from build123d import *

# Parameters (mm, degrees)
CYLINDER002_R       = 3.8
CYLINDER002_DEPTH   = 15
CYLINDER001_R       = 2
CYLINDER001_DEPTH   = 16
BOX001_W            = 5
BOX001_H            = 20
BOX001_DEPTH        = 12
BOX_W               = 5
BOX_H               = 20
BOX_DEPTH           = 12
BOX_PLACEMENT_ANGLE = 90
CYLINDER_R          = 10
CYLINDER_DEPTH      = 16


with BuildPart() as cilindro002:
    # Cylinder002 → Cylinder002 (new body)
    with BuildSketch(Plane.XY):
        Circle(CYLINDER002_R)
    extrude(amount=CYLINDER002_DEPTH)


with BuildPart() as fusion001:
    # Cylinder001 → Cylinder001 (new body)
    with BuildSketch(Plane.XY):
        Circle(CYLINDER001_R)
    extrude(amount=CYLINDER001_DEPTH)

    # Fusion001: union Cilindro002
    add(cilindro002.part)


with BuildPart() as cubo001:
    # Box001 → Box001 (new body)
    with BuildSketch(Plane(origin=(-2.5, -10, 0), x_dir=(1, 0, 0), z_dir=(0, 0, 1))):
        with Locations((2.5, 10)):
            Rectangle(BOX001_W, BOX001_H)
    extrude(amount=BOX001_DEPTH)


with BuildPart() as fusion:
    # Box → Box (new body)
    with BuildSketch(Plane.XY):
        with Locations((2.5, 10)):
            Rectangle(BOX_W, BOX_H)
    extrude(amount=BOX_DEPTH)


with BuildPart() as fusion_1:
    # Box placement: moved
    add(fusion.part.moved(Location((10, -2.5, 0))).rotate(Axis((10, -2.5, 0), (0, 0, 1)), BOX_PLACEMENT_ANGLE))

    # Fusion: union Cubo001
    add(cubo001.part)


with BuildPart() as esfera:
    # Sphere → Sphere (revolve)
    with BuildSketch(Plane(origin=(0, 0, 3), x_dir=(1, 0, 0), z_dir=(0, -1, 0))):
        with BuildLine():
            ThreePointArc((0, -8), (8, 0), (0, 8))
            Line((0, 8), (0, -8))
        make_face()
    revolve(axis=Axis((0, 0, 3), (0, 0, 1)))


with BuildPart() as cut002:
    # Cylinder → Cylinder (new body)
    with BuildSketch(Plane.XY):
        Circle(CYLINDER_R)
    extrude(amount=CYLINDER_DEPTH)

    # Cut: cut Esfera
    add(esfera.part, mode=Mode.SUBTRACT)

    # Cut001: cut Fusion
    add(fusion_1.part, mode=Mode.SUBTRACT)

    # Cut002: cut Fusion001
    add(fusion001.part, mode=Mode.SUBTRACT)


solid = cut002.part
Read the model definition and answer for the solid it produces. Units are mm, in the model's axes. A direction names the side the tool comes from. Round coordinates to 2 decimals unless told otherwise and drop trailing zeros. Loops run counter-clockwise (first coordinate to the right, second up) from the corner with the lowest first, then second, coordinate; pieces in that order, holes last.
Q1. Which of the six approach directions +Z, -Z, +X, -X, +Y, -Y give full straight-line access (tool end or side, diameter ignored) to faces 1 (the face through (-6, 6, 0)), 2 (the face through (-7, -2.5, 7)), 3 (the face through (2, -2, 15)), 4 (the face through (2.5, -7, 7))?
Q2. Determine the mould class of faces 5 (the face through (-7, 2.5, 7)), 6 (the face through (-2.5, 7, 7)), 7 (the face through (2.5, 7, 7)), 8 (the face through (9.237, -3.83, 7.888)) for opening direction X: released by +X, released by -X, zero draft, split by the parting line, or undercut.
Q3. Each of these flat-tipped pins is pushed along its axis until it touches: pin 1 (4 mm diameter, centred on x = 2.5, z = 14, fed in from -Y); pin 2 (5.5 mm diameter, centred on y = -7.5, z = 8, fed in from -X); pin 3 (7 mm diameter, centred on x = 0, y = 0, fed in from -Z). Where does it stop, or does it pass through?
Q4. Section A-A on z = 11 is taken. Write down the section's boundary in (x, y).
Q5. Consider probe 1 along Y at (x, z) = (0, 15.65); probe 2 along Y at (x, z) = (0, 12.3). Determine where each line is inside the solid, lowest interval first.
Q6. Section D-D on z = 8.5 is taken. Write down the section's boundary in (x, y).
Q7. Section B-B on x = 0 is taken. Write down the section's boundary in (y, z), and give its area (3 significant figures).
Output:
1. face 1: -Z, +X, -X, +Y, -Y
1. face 2: -Z, +X, -X
1. face 3: -Z
1. face 4: -Z, +Y, -Y
2. face 5: zero draft
2. face 6: undercut
2. face 7: undercut
2. face 8: split by the parting line
3. pin 1: stops at y = -9.99
3. pin 2: stops at x = -8.8
3. pin 3: stops at z = 15
4. outline: (-9.68, -2.5) arc R10 ccw to (-2.5, -9.68) - (-2.5, -2.86) arc R3.8 cw to (-2.86, -2.5) - close; (-9.68, 2.5) - (-2.86, 2.5) arc R3.8 cw to (-2.5, 2.86) - (-2.5, 9.68) arc R10 ccw to start; (2.5, -9.68) arc R10 ccw to (9.68, -2.5) - (2.86, -2.5) arc R3.8 cw to (2.5, -2.86) - close; (2.5, 2.86) arc R3.8 cw to (2.86, 2.5) - (9.68, 2.5) arc R10 ccw to (2.5, 9.68) - close
5. probe 1: y = -10 to -2, 2 to 10
5. probe 2: y = -10 to -3.8, 3.8 to 10
6. outline: (-9.68, -2.5) arc R10 ccw to (-2.5, -9.68) - (-2.5, -5.24) arc R5.81 cw to (-5.24, -2.5) - close; (-9.68, 2.5) - (-5.24, 2.5) arc R5.81 cw to (-2.5, 5.24) - (-2.5, 9.68) arc R10 ccw to start; (2.5, -9.68) arc R10 ccw to (9.68, -2.5) - (5.24, -2.5) arc R5.81 cw to (2.5, -5.24) - close; (2.5, 5.24) arc R5.81 cw to (5.24, 2.5) - (9.68, 2.5) arc R10 ccw to (2.5, 9.68) - close
7. outline: (-10, 12) - (-3.8, 12) - (-3.8, 15) - (-2, 15) - (-2, 16) - (-10, 16) - close; (2, 15) - (3.8, 15) - (3.8, 12) - (10, 12) - (10, 16) - (2, 16) - close
7. area: 53.2 mm2
